Can you work these out from the model? Positions are in its coordinate system, mm. A direction names the side the tool comes from. Round coordinates to 2 decimals unless told otherwise and drop trailing zeros. One line per question, with ' | ' between items.
```python
from build123d import *


with BuildPart() as f2:
    # F2: sweep along a path in F1
    with BuildLine(Plane.YZ) as f2_path:
        Line((0, 0), (0, 30))
        Line((0, 30), (-20.5212085995, 86.3815572472))
        Line((-20.5212085995, 86.3815572472), (-50.5212085995, 122.134165025))
    # F0 (on Top) → F2 (sweep)
    with BuildSketch(Plane.XY):
        with BuildLine():
            Line((-14, -15), (14, -15))
            ThreePointArc((14, -15), (18.2426406871, -13.2426406871), (20, -9))
            Line((20, -9), (20, 9))
            ThreePointArc((20, 9), (18.2426406871, 13.2426406871), (14, 15))
            Line((14, 15), (4, 15))
            Line((4, 15), (4, 2.1593614055))
            add(Edge.make_bspline(
                [(-4, 2.1593614055), (-27.382723871, -0.1854807252), (-13.6913619355, -8.2115012982), (0, -16.2375218712), (13.6913619355, -8.2115012982), (27.382723871, -0.1854807252), (4, 2.1593614055)],
                knots=[4.9551445309, 4.9551445309, 4.9551445309, 6.8877025996, 6.8877025996, 8.8202606683, 8.8202606683, 10.752818737, 10.752818737, 10.752818737], degree=2, weights=[1, 0.568364982, 1, 0.568364982, 1, 0.568364982, 1]))
            Line((-4, 2.1593614055), (-4, 15))
            Line((-4, 15), (-14, 15))
            ThreePointArc((-14, 15), (-18.2426406871, 13.2426406871), (-20, 9))
            Line((-20, 9), (-20, -9))
            ThreePointArc((-20, -9), (-18.2426406871, -13.2426406871), (-14, -15))
        make_face()
    sweep(path=f2_path.line, transition=Transition.RIGHT)


solid = f2.part
```
(1) Will these pins go through, and if not, where does the flat tip stop? pin 1 Ø12 at (x, y) = (15, -45) entering from +Z; pin 2 Ø6 at (x, z) = (3, 20.5) entering from -Y; pin 3 Ø22 at (x, z) = (6, 19) entering from -Y.
Final values:
pin 1: z = 131.77 | pin 2: y = -15 | pin 3: y = -15.96
(2) On a 3-axis mill with a long thin cutter (end or side, diameter ignored), from which of +Z, -Z, +X, -X, +Y, -Y can I reach the whole of each face in a straight line? I mean faces 4 (the cylindrical face through (-18.289, -13.196, 14.405)), 5 (the cylindrical face through (18.196, -13.289, 14.405)), 6 (the cylindrical face through (18.289, 13.196, 16.551)). Say none if no direction works.
Final values:
face 4: -Z, -X, -Y | face 5: -Z, +X, -Y | face 6: +Z, -Z, +X, +Y
(3) Thinking about a two-plate mould opening in X: for faces 1 (the cylindrical face through (-18.196, -24.713, 112.051)), 2 (the cylindrical face through (18.2, -46.41, 96.57)), 3 (the flat face through (4, -10, 66)), which applies, released by +X, released by -X, zero draft, split by the parting line, or undercut?
Final values:
face 1: released by -X | face 2: released by +X | face 3: undercut
(4) Please list where these lines run through material, in increasing order: probe 1 along X at (y, z) = (-18.5, 92); probe 2 along Y at (x, z) = (7, 51); probe 3 along Z at (x, y) = (10, -40). Write a range as [from, to].
Final values:
probe 1: [-20, -4], [4, 20] | probe 2: [-23.61, -18.81], [-5.8, 8.32] | probe 3: [86.26, 94.4], [111.16, 130.96]
